from build123d import *

# Parameters (mm, degrees)
SKETCH_R     = 1.5
SKETCH_R_2   = 6
PAD_DEPTH    = 5
POCKET_DEPTH = 2
FILLET_R     = 2


with BuildPart() as part:
    # Sketch → Pad (new body)
    with BuildSketch(Plane.XY):
        with BuildLine():
            Line((-15, -3), (-5, -3))
            Line((-5, -3), (-5, -14.202041))
            ThreePointArc((-5, -14.202041), (0, -35), (5, -14.202041))
            Line((5, -14.202041), (5, -3))
            Line((5, -3), (15, -3))
            Line((15, -3), (15, 3))
            Line((15, 3), (-15, 3))
            Line((-15, 3), (-15, -3))
        make_face()
        with Locations((11.5, 0)):
            Circle(SKETCH_R, mode=Mode.SUBTRACT)
        with Locations((-11.5, 0)):
            Circle(SKETCH_R, mode=Mode.SUBTRACT)
        with Locations((0, -24)):
            Circle(SKETCH_R_2, mode=Mode.SUBTRACT)
    extrude(amount=PAD_DEPTH)

    # Sketch001 → Pocket (cut)
    with BuildSketch(Plane.XY.offset(5)):
        Polygon((4.87861, -32.45), (9.75722, -24), (4.87861, -15.55), (-4.87861, -15.55), (-9.75722, -24), (-4.87861, -32.45), align=None)
    extrude(amount=-POCKET_DEPTH, mode=Mode.SUBTRACT)

    # Fillet
    fillet_edges = [part.edges().sort_by_distance(p)[0] for p in [
        (15, 3, 2.5),
        (15, -3, 2.5),
        (-15, 3, 2.5),
        (-15, -3, 2.5),
        (-5, -3, 2.5),
        (5, -3, 2.5),
        (5, -14.202041, 2.5),
        (-5, -14.202041, 2.5),
    ]]
    fillet(fillet_edges, radius=FILLET_R)


solid = part.part
Could you check a few things on this model? Use its own coordinates, in mm. A direction names the side the tool comes from. Give positions to 0.01 mm unless a question says otherwise; leave off trailing zeros. Order: outer loops, then holes, each group sorted by start corner. A loop starts at its lowest first (then second) coordinate and runs counter-clockwise, first axis right, second up.
Item 1: I'm going to push flat-ended pins straight in: pin 1 (5 mm diameter, centred on x = -11.5, y = 0, fed in from +Z); pin 2 (1.6 mm diameter, centred on x = 2, z = 3.5, fed in from -Y); pin 3 (1.8 mm diameter, centred on x = 11.5, y = 0, fed in from -Z); pin 4 (3 mm diameter, centred on y = -12, z = 1, fed in from +X). Where does each tip first touch, or does it pass through?
Item 2: If we section it at C-C, the plane z = 4: Write out the boundary of the cut face in (x, y).
Item 3: If we section it at D-D, the plane y = -22: Write out the boundary of the cut face in (x, z).
Item 4: If we section it at B-B, the plane y = 0: Write out the boundary of the cut face in (x, z), plus the area to 3 significant figures.
Item 5: If we section it at A-A, the plane x = 0: Write out the boundary of the cut face in (y, z), plus the area to 3 significant figures.
Item 6: If we mould it in two halves opening along Y, with no side actions, what happens to faces 4 (the face through (-14.43, 2.4, 2.54)), 5 (the face through (-10, -3, 2)), 6 (the face through (5.253, -14.019, 2.535)), 7 (the face through (-14.4, -2.43, 2.54))? For each: pulls with the +Y half, pulls with the -Y half, needs draft (parallel to the pull), parting line crosses it, or undercut.
Item 7: I need wall thicknesses on line 1 (Y direction, x = -11.5, z = 1.55); line 2 (Y direction, x = -7.75, z = 3.6); line 3 (Y direction, x = 7.5, z = 4.2). Which ranges of each line are inside material? Lowest first, please.
Item 8: For faces 1 (the face through (-5, -9, 2)), 2 (the face through (2, -18, 3)), 3 (the face through (5, -9, 2)), which set-ups out of +Z, -Z, +X, -X, +Y, -Y let a thin tool reach every point of the face, with its end or its side?
Values:
1. pin 1: stops at z = 5
1. pin 2: stops at y = -34.93
1. pin 3: passes through
1. pin 4: stops at x = 5.05
2. outline: (-15, -1) arc R2 ccw to (-13, -3) - (-7, -3) arc R2 cw to (-5, -5) - (-5, -13.05) arc R2 cw to (-5.92, -14.73) arc R11 ccw (long way) to (5.92, -14.73) arc R2 cw to (5, -13.05) - (5, -5) arc R2 cw to (7, -3) - (13, -3) arc R2 ccw to (15, -1) - (15, 1) arc R2 ccw to (13, 3) - (-13, 3) arc R2 ccw to (-15, 1) - close; hole circle Ø3 at (-11.5, 0); hole (-9.76, -24) - (-4.88, -32.45) - (4.88, -32.45) - (9.76, -24) - (4.88, -15.55) - (-4.88, -15.55) - close; hole circle Ø3 at (11.5, 0)
3. outline: (-10.82, 0) - (-5.66, 0) - (-5.66, 3) - (-8.6, 3) - (-8.6, 5) - (-10.82, 5) - close; (5.66, 0) - (10.82, 0) - (10.82, 5) - (8.6, 5) - (8.6, 3) - (5.66, 3) - close
4. outline: (-15, 0) - (-13, 0) - (-13, 5) - (-15, 5) - close; (-10, 0) - (10, 0) - (10, 5) - (-10, 5) - close; (13, 0) - (15, 0) - (15, 5) - (13, 5) - close
4. area: 120 mm2
5. outline: (-35, 0) - (-30, 0) - (-30, 3) - (-32.45, 3) - (-32.45, 5) - (-35, 5) - close; (-18, 0) - (3, 0) - (3, 5) - (-15.55, 5) - (-15.55, 3) - (-18, 3) - close
5. area: 120 mm2
6. face 4: pulls with the +Y half
6. face 5: undercut
6. face 6: undercut
6. face 7: pulls with the -Y half
7. line 1: y = -3 to -1.5, 1.5 to 3
7. line 2: y = -31.81 to -27.48, -20.52 to -16.19, -3 to 3
7. line 3: y = -32.05 to -27.91, -20.09 to -15.95, -3 to 3
8. face 1: +Z, -Z, -X
8. face 2: +Z
8. face 3: +Z, -Z, +X
